Answer from the drawing. Dimensions are ordinates in mm from the lowest x, y and z of the part. Give positions to 0.01 mm unless a question says otherwise; leave off trailing zeros. Loops run counter-clockwise (first coordinate to the right, second up) from the corner with the lowest first, then second, coordinate; pieces in that order, holes last. Notation, with made-up numbers: M -19.5,72 L 29.5,72 A35 cw 29.5,107 Z; hole C 78.5,62 d4. An arc over 180 degrees is marked long. Return JSON: item names as keys, results as strings. Group by question number.
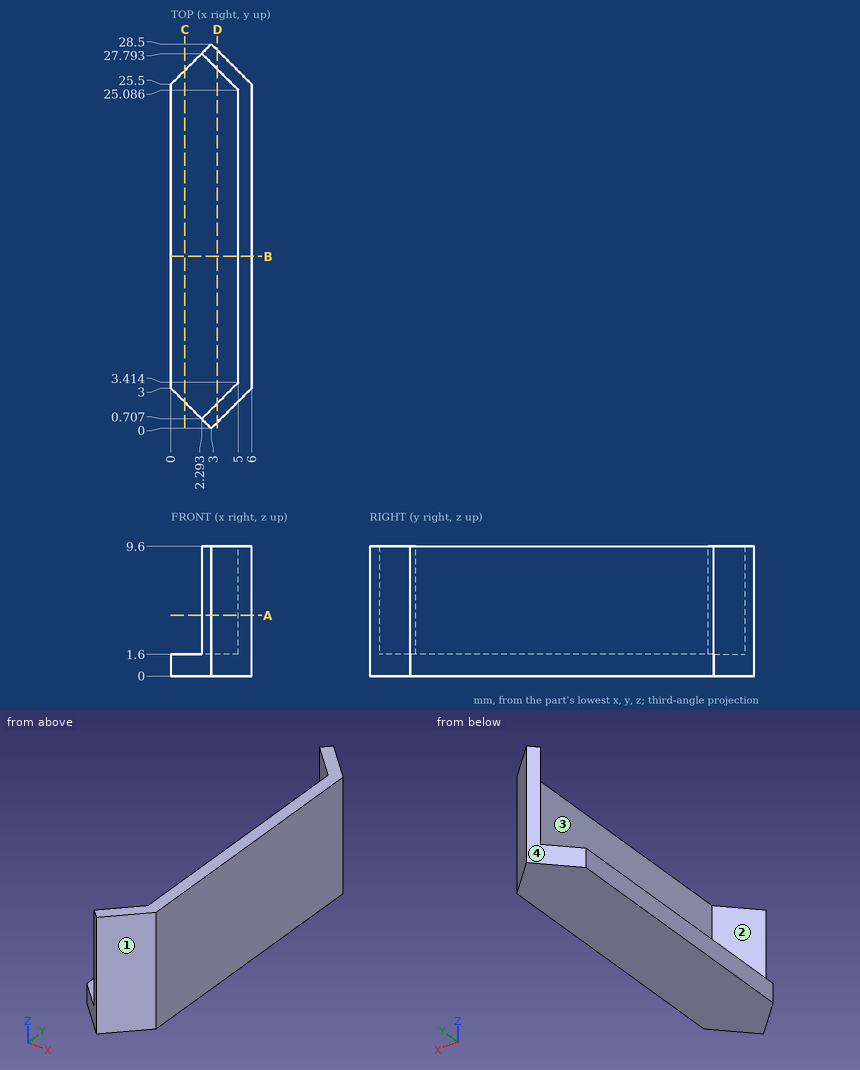
1. Flat-ended cylindrical pins translate along their axes: P1, Ø4, axis at y = 14.5, z = 7, coming from the -X side; P2, Ø2.5, axis at x = 3, y = 11.5, coming from the +Z side. Find the tip coordinate at first contact, or state that the pin passes through.
2. Find section C-C (x = 1.05). Write down the section's boundary in (y, z).
3. Straight lines are drawn through the part: line 1 along Z through (x, y) = (3.55, 7); line 2 along X through (y, z) = (18.5, 9.25); line 3 along Y through (x, z) = (3.7, 4.5) (1 decimal). For each, find the intervals that lie inside material, in ascending order.
4. Find section B-B (y = 12.75). Write down the section's boundary in (x, z), and give its area (3 significant figures).
5. Find section A-A (z = 4.5). Write down the section's boundary in (x, y).
6. The mould has two halves that part along Y. Classify the marked faces 1, 2, 3 and 4: +Y half, -Y half, draft (parallel to the pull), parting line (faces both ways), or undercut.
7. Find section D-D (x = 3.45). Write down the section's boundary in (y, z).
Result:
{
 "1": {"P1": "stops at x = 5", "P2": "stops at z = 1.6"},
 "2": {"outline": "M 1.95,0 L 26.55,0 L 26.55,1.6 L 1.95,1.6 Z"},
 "3": {"line 1": "z = 0 to 1.6", "line 2": "x = 5 to 6", "line 3": "y = 0.7 to 2.1, 26.4 to 27.8"},
 "4": {"outline": "M 0,0 L 6,0 L 6,9.6 L 5,9.6 L 5,1.6 L 0,1.6 Z", "area": "17.6 mm2"},
 "5": {"outline": "M 2.29,0.71 L 3,0 L 6,3 L 6,25.5 L 3,28.5 L 2.29,27.79 L 5,25.09 L 5,3.41 Z"},
 "6": {"face 1": "-Y half", "face 2": "undercut", "face 3": "undercut", "face 4": "+Y half"},
 "7": {"outline": "M 0.45,0 L 28.05,0 L 28.05,9.6 L 26.64,9.6 L 26.64,1.6 L 1.86,1.6 L 1.86,9.6 L 0.45,9.6 Z"}
}
